Part model, mm, in its own coordinate system. Face numbers are marked on the shaded views. A direction names the side the tool comes from. Coordinates: 2 decimals unless noted, no trailing zeros. Order: outer loops, then holes, each group sorted by start corner. A loop starts at its lowest first (then second) coordinate and runs counter-clockwise, first axis right, second up.
1) Cut at C-C (z = 24.5). List the corners of the cut face in (x, y).
2) Mould opens along X. For the marked faces 1 and 2 say: +X half, -X half, draft (parallel to the pull), parting line (faces both ways), or undercut.
3) Pin check, flat tips, straight feed: pin 1 Ø5.5 at (x, z) = (-32, -15.5) entering from +Y; pin 2 Ø4 at (x, y) = (-44, 10.5) entering from -Z; pin 3 Ø10 at (x, z) = (14, 35.5) entering from +Y; pin 4 Ø24 at (x, z) = (8.5, 0) entering from -Y. Stop position of each tip, or through.
4) Cut at A-A (z = 0). List the corners of the cut face in (x, y), and give its area (3 significant figures).
5) Tool access for the marked faces 3, 4 and 5: list every direction of +Z, -Z, +X, -X, +Y, -Y with a clear straight run to the whole face (end or side of a thin tool).
6) Wall check: L1, parallel to X at y = -7.25, z = 0; L2, parallel to Z at x = -31.5, y = -5.5; L3, parallel to Z at x = 3.5, y = -9. Give the ranges that are in metal, low to high.
7) Cut at D-D (x = 15). List the corners of the cut face in (y, z).
8) Cut at B-B (x = 0). List the corners of the cut face in (y, z), and give its area (3 significant figures).
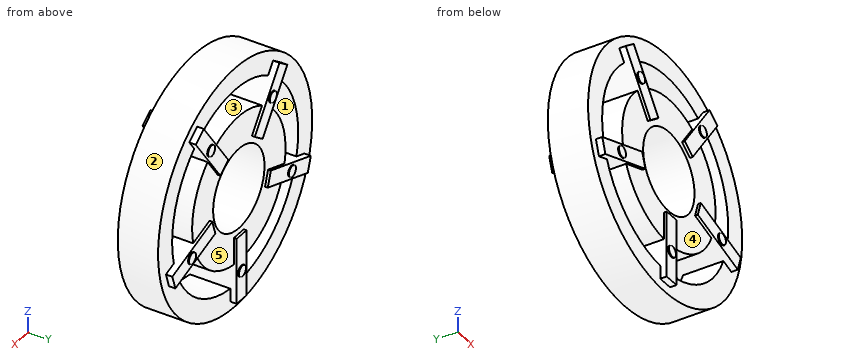
```python
from build123d import *

# Parameters (mm, degrees)
SKETCH1_R            = 66
SKETCH1_R_2          = 54
RIM_OUTER_RING_DEPTH = 11
SKETCH2_R            = 40
SKETCH2_R_2          = 22
RIM_HUB_RING_DEPTH   = 13
RIM_SPOKE_1_DEPTH    = 14.5
SKETCH4_R            = 3
RIM_BOLT_PAD_1_DEPTH = 15
SKETCH5_W            = 8.4
SKETCH5_H            = 36
RIM_SPOKE_2_DEPTH    = 14.5
SKETCH6_R            = 3
RIM_BOLT_PAD_2_DEPTH = 15
RIM_SPOKE_3_DEPTH    = 14.5
SKETCH8_R            = 3
RIM_BOLT_PAD_3_DEPTH = 15
RIM_SPOKE_4_DEPTH    = 14.5
SKETCH10_R           = 3
RIM_BOLT_PAD_4_DEPTH = 15
RIM_SPOKE_5_DEPTH    = 14.5
SKETCH12_R           = 3
RIM_BOLT_PAD_5_DEPTH = 15


with BuildPart() as part:
    # Sketch1 → rim outer ring (new, symmetric)
    with BuildSketch(Plane(origin=(0, 0, 0), x_dir=(1, 0, 0), z_dir=(0, 1, 0))):
        with Locations(Location((0, 0, 0), (0, 0, 270))):
            Circle(SKETCH1_R)
        with Locations(Location((0, 0, 0), (0, 0, 270))):
            Circle(SKETCH1_R_2, mode=Mode.SUBTRACT)
    extrude(amount=RIM_OUTER_RING_DEPTH, both=True)



with BuildPart() as body_2:
    # Sketch2 → rim hub ring (new, symmetric)
    with BuildSketch(Plane(origin=(0, 0, 0), x_dir=(1, 0, 0), z_dir=(0, 1, 0))):
        with Locations(Location((0, 0, 0), (0, 0, 90))):
            Circle(SKETCH2_R)
        with Locations(Location((0, 0, 0), (0, 0, 90))):
            Circle(SKETCH2_R_2, mode=Mode.SUBTRACT)
    extrude(amount=RIM_HUB_RING_DEPTH, both=True)


with BuildPart() as part_1:
    add(part.part)

    add(body_2.part)  # rim spoke 1 merges body 2
    # Sketch3 → rim spoke 1 (add, symmetric)
    with BuildSketch(Plane(origin=(0, 0, 0), x_dir=(1, 0, 0), z_dir=(0, 1, 0))):
        Polygon((22.478541531, 11.719862228), (56.716576118, 22.844474025), (59.31231887, 14.855599288), (25.074284284, 3.730987491), align=None)
    extrude(amount=RIM_SPOKE_1_DEPTH, both=True)

    # Sketch4 → rim bolt pad 1 (add, symmetric)
    with BuildSketch(Plane(origin=(0, 0, 0), x_dir=(1, 0, 0), z_dir=(0, 1, 0))):
        with Locations(Location((42.797543233, 13.905764747, 0), (0, 0, 90))):
            Circle(SKETCH4_R)
    extrude(amount=RIM_BOLT_PAD_1_DEPTH, both=True)

    # Sketch5 → rim spoke 2 (add, symmetric)
    with BuildSketch(Plane(origin=(0, 0, 0), x_dir=(1, 0, 0), z_dir=(0, 1, 0))):
        with Locations((0, 43)):
            Rectangle(SKETCH5_W, SKETCH5_H)
    extrude(amount=RIM_SPOKE_2_DEPTH, both=True)

    # Sketch6 → rim bolt pad 2 (add, symmetric)
    with BuildSketch(Plane(origin=(0, 0, 0), x_dir=(1, 0, 0), z_dir=(0, 1, 0))):
        with Locations(Location((0, 45, 0), (0, 0, 90))):
            Circle(SKETCH6_R)
    extrude(amount=RIM_BOLT_PAD_2_DEPTH, both=True)

    # Sketch7 → rim spoke 3 (add, symmetric)
    with BuildSketch(Plane(origin=(0, 0, 0), x_dir=(1, 0, 0), z_dir=(0, 1, 0))):
        Polygon((-25.074284284, 3.730987491), (-59.31231887, 14.855599288), (-56.716576118, 22.844474025), (-22.478541531, 11.719862228), align=None)
    extrude(amount=RIM_SPOKE_3_DEPTH, both=True)

    # Sketch8 → rim bolt pad 3 (add, symmetric)
    with BuildSketch(Plane(origin=(0, 0, 0), x_dir=(1, 0, 0), z_dir=(0, 1, 0))):
        with Locations(Location((-42.797543233, 13.905764747, 0), (0, 0, 90))):
            Circle(SKETCH8_R)
    extrude(amount=RIM_BOLT_PAD_3_DEPTH, both=True)

    # Sketch9 → rim spoke 4 (add, symmetric)
    with BuildSketch(Plane(origin=(0, 0, 0), x_dir=(1, 0, 0), z_dir=(0, 1, 0))):
        Polygon((-11.296759931, -22.694122919), (-32.457029013, -51.818734717), (-39.252771766, -46.881338597), (-18.092502684, -17.7567268), align=None)
    extrude(amount=RIM_SPOKE_4_DEPTH, both=True)

    # Sketch10 → rim bolt pad 4 (add, symmetric)
    with BuildSketch(Plane(origin=(0, 0, 0), x_dir=(1, 0, 0), z_dir=(0, 1, 0))):
        with Locations(Location((-26.450336353, -36.405764747, 0), (0, 0, 90))):
            Circle(SKETCH10_R)
    extrude(amount=RIM_BOLT_PAD_4_DEPTH, both=True)

    # Sketch11 → rim spoke 5 (add, symmetric)
    with BuildSketch(Plane(origin=(0, 0, 0), x_dir=(1, 0, 0), z_dir=(0, 1, 0))):
        Polygon((18.092502684, -17.7567268), (39.252771766, -46.881338597), (32.457029013, -51.818734717), (11.296759931, -22.694122919), align=None)
    extrude(amount=RIM_SPOKE_5_DEPTH, both=True)

    # Sketch12 → rim bolt pad 5 (add, symmetric)
    with BuildSketch(Plane(origin=(0, 0, 0), x_dir=(1, 0, 0), z_dir=(0, 1, 0))):
        with Locations(Location((26.450336353, -36.405764747, 0), (0, 0, 90))):
            Circle(SKETCH12_R)
    extrude(amount=RIM_BOLT_PAD_5_DEPTH, both=True)


solid = part_1.part
```
Geometry check:
1. outline: (-61.28, -11) - (-48.12, -11) - (-48.12, 11) - (-61.28, 11) - close; (-31.62, -13) - (-22.99, -13) - (-22.99, -14.5) - (-12.61, -14.5) - (-12.61, -13) - (12.61, -13) - (12.61, -14.5) - (22.99, -14.5) - (22.99, -13) - (31.62, -13) - (31.62, 13) - (22.99, 13) - (22.99, 14.5) - (12.61, 14.5) - (12.61, 13) - (-12.61, 13) - (-12.61, 14.5) - (-22.99, 14.5) - (-22.99, 13) - (-31.62, 13) - close; (48.12, -11) - (61.28, -11) - (61.28, 11) - (48.12, 11) - close
2. face 1: undercut
2. face 2: parting line
3. pin 1: stops at y = 14.5
3. pin 2: stops at z = -50.91
3. pin 3: stops at y = 13
3. pin 4: passes through
4. outline: (-66, -11) - (-54, -11) - (-54, 11) - (-66, 11) - close; (-40, -13) - (-22, -13) - (-22, 13) - (-40, 13) - close; (22, -13) - (40, -13) - (40, 13) - (22, 13) - close; (54, -11) - (66, -11) - (66, 11) - (54, 11) - close
4. area: 1,460 mm2
5. face 3: +Y, -Y
5. face 4: -Y
5. face 5: +Y
6. L1: x = -66 to -54, -40 to -22, 22 to 40, 54 to 66
6. L2: z = -58 to -43.86, -24.65 to 24.65, 36.21 to 58
6. L3: z = -65.91 to -21.72, 21.72 to 39.85, 53.89 to 65.91
7. outline: (-14.5, 20) - (-13, 20) - (-13, 16.09) - (13, 16.09) - (13, 20) - (14.5, 20) - (14.5, 27.79) - (13, 27.79) - (13, 37.08) - (-13, 37.08) - (-13, 27.79) - (-14.5, 27.79) - close; (-13, -37.08) - (13, -37.08) - (13, -16.09) - (-13, -16.09) - close; (-11, -64.27) - (11, -64.27) - (11, -51.87) - (-11, -51.87) - close; (-11, 51.87) - (11, 51.87) - (11, 64.27) - (-11, 64.27) - close
8. outline: (-15, -48) - (-14.5, -48) - (-14.5, -61) - (-11, -61) - (-11, -66) - (11, -66) - (11, -61) - (14.5, -61) - (14.5, -48) - (15, -48) - (15, -42) - (14.5, -42) - (14.5, -25) - (13, -25) - (13, -22) - (-13, -22) - (-13, -25) - (-14.5, -25) - (-14.5, -42) - (-15, -42) - close; (-13, 22) - (13, 22) - (13, 40) - (-13, 40) - close; (-11, 54) - (11, 54) - (11, 66) - (-11, 66) - close
8. area: 1,970 mm2
